Here's how the part is built. I have some questions about the finished solid (model axes, mm). Round coordinates to 2 decimals unless told otherwise and drop trailing zeros. Write each loop counter-clockwise with the first axis right and the second up, starting at its lowest first coordinate (ties: lowest second). Pieces come first, ordered by that corner, then holes. Notation, with made-up numbers: (5, 34) - (27, 34) arc R23 cw to (27, 57) - close; hole circle Ø1 at (34.25, -11.75). An arc over 180 degrees is marked (long way). Use one line per item in the form item = value. Start each with the question number.
1. I want a section at A-A, the plane x = 134.25. List the corners of the cut face in (y, z) for me.
2. I want a section at C-C, the plane x = 57.9. List the corners of the cut face in (y, z) for me, plus the area to 3 significant figures.
3. I want a section at D-D, the plane z = 4.15. List the corners of the cut face in (x, y) for me, plus the area to 3 significant figures.
4. I want a section at B-B, the plane y = 6.85. List the corners of the cut face in (x, z) for me, plus the area to 3 significant figures.
5. Will these pins go through, and if not, where does the flat tip stop? pin 1 (6 mm diameter, centred on x = 57.9, y = 6.85, fed in from +Z); pin 2 (8 mm diameter, centred on x = 137, y = 17.5, fed in from -Z).
6. If I drill on line 1 along X through (y, z) = (7, 2.75); line 2 along Y through (x, z) = (99.1, 3.6); line 3 along X through (y, z) = (18.5, 3.55), over which ranges is the centre line in solid material (lowest first)?
7. We'd pull the mould along X, two halves only. Please class faces 1 (the cylindrical face through (59.655, 6.122, 2.504)), 2 (the cylindrical face through (155.859, 38.797, 2.504)), 3 (the flat face through (77, 0, 3)), 4 (the cylindrical face through (1.203, 38.859, 2.504)): +X half, -X half, draft (parallel to the pull), parting line (faces both ways), or undercut.
```python
from build123d import *

# Parameters (mm, degrees)
F0_R     = 1.9
F0_R_2   = 7.75
F1_DEPTH = 5.08


with BuildPart() as f1:
    # F0 (on Top) → F1 (new body)
    with BuildSketch(Plane.XY):
        with BuildLine():
            ThreePointArc((0, 4), (1.171573, 1.171573), (4, 0))
            Line((4, 0), (153, 0))
            ThreePointArc((153, 0), (155.828427, 1.171573), (157, 4))
            Line((157, 4), (157, 36))
            ThreePointArc((157, 36), (155.828427, 38.828427), (153, 40))
            Line((153, 40), (4, 40))
            ThreePointArc((4, 40), (1.171573, 38.828427), (0, 36))
            Line((0, 36), (0, 4))
        make_face()
        with Locations((57.9, 6.85)):
            Circle(F0_R, mode=Mode.SUBTRACT)
        with Locations((99.1, 6.85)):
            Circle(F0_R, mode=Mode.SUBTRACT)
        with Locations((22.75, 20)):
            Circle(F0_R_2, mode=Mode.SUBTRACT)
        with Locations((57.9, 33.15)):
            Circle(F0_R, mode=Mode.SUBTRACT)
        with Locations((78.5, 20)):
            Circle(F0_R_2, mode=Mode.SUBTRACT)
        with Locations((134.25, 20)):
            Circle(F0_R_2, mode=Mode.SUBTRACT)
        with Locations((99.1, 33.15)):
            Circle(F0_R, mode=Mode.SUBTRACT)
    extrude(amount=F1_DEPTH)


solid = f1.part
```
Model answer:
q1.outline = (0, 0) - (12.25, 0) - (12.25, 5.08) - (0, 5.08) - close; (27.75, 0) - (40, 0) - (40, 5.08) - (27.75, 5.08) - close
q2.outline = (0, 0) - (4.95, 0) - (4.95, 5.08) - (0, 5.08) - close; (8.75, 0) - (31.25, 0) - (31.25, 5.08) - (8.75, 5.08) - close; (35.05, 0) - (40, 0) - (40, 5.08) - (35.05, 5.08) - close
q2.area = 165 mm2
q3.outline = (0, 4) arc R4 ccw to (4, 0) - (153, 0) arc R4 ccw to (157, 4) - (157, 36) arc R4 ccw to (153, 40) - (4, 40) arc R4 ccw to (0, 36) - close; hole circle Ø15.5 at (22.75, 20); hole circle Ø3.8 at (57.9, 6.85); hole circle Ø3.8 at (57.9, 33.15); hole circle Ø15.5 at (78.5, 20); hole circle Ø3.8 at (99.1, 6.85); hole circle Ø3.8 at (99.1, 33.15); hole circle Ø15.5 at (134.25, 20)
q3.area = 5,650 mm2
q4.outline = (0, 0) - (56, 0) - (56, 5.08) - (0, 5.08) - close; (59.8, 0) - (97.2, 0) - (97.2, 5.08) - (59.8, 5.08) - close; (101, 0) - (157, 0) - (157, 5.08) - (101, 5.08) - close
q4.area = 759 mm2
q5.pin_1 = 5.08
q5.pin_2 = through
q6.line_1 = 0 to 56.01, 59.79 to 97.21, 100.99 to 157
q6.line_2 = 0 to 4.95, 8.75 to 31.25, 35.05 to 40
q6.line_3 = 0 to 15.15, 30.35 to 70.9, 86.1 to 126.65, 141.85 to 157
q7.face_1 = undercut
q7.face_2 = +X half
q7.face_3 = draft
q7.face_4 = -X half
